Read the model definition and answer for the solid it produces. Units are mm, in the model's axes. Face numbers are marked on the shaded views. A direction names the side the tool comes from. Give positions to 0.01 mm unless a question says otherwise; leave off trailing zeros. Order: outer loops, then holes, each group sorted by start corner. A loop starts at its lowest first (then second) coordinate and runs counter-clockwise, first axis right, second up.
Item 1: A cutting plane is placed at B-B (y = 9.5). Write down the section's boundary in (x, z).
Item 2: A cutting plane is placed at A-A (x = 0). Write down the section's boundary in (y, z).
Item 3: The mould has two halves that part along X. Classify the marked faces 1 and 2: +X half, -X half, draft (parallel to the pull), parting line (faces both ways), or undercut.
Item 4: Find the intervals of material crossed by line 1 along Y through (x, z) = (0, 7.25); line 2 along X through (y, z) = (18.5, 7.75); line 3 along Y through (x, z) = (-77.5, 7.5), in increasing order.
Item 5: A cutting plane is placed at C-C (x = -61.5). Write down the section's boundary in (y, z).
Item 6: Given pin 1 Ø1 at (y, z) = (18.5, 1.5) entering from +X; pin 2 Ø1.5 at (x, z) = (-64.5, 6) entering from +Y; pin 3 Ø6 at (x, y) = (-5, 21.5) entering from -Z; pin 4 Ø6 at (x, y) = (-24.5, 15) entering from +Z, each flat-ended and moving along its own axis, determine where each tip first touches the part or whether it passes through.
Item 7: Which of the six approach directions +Z, -Z, +X, -X, +Y, -Y give full straight-line access (tool end or side, diameter ignored) to the marked faces 3 and 4?
Item 8: A cutting plane is placed at D-D (x = -104.5). Write down the section's boundary in (y, z), plus the area to 3 significant figures.
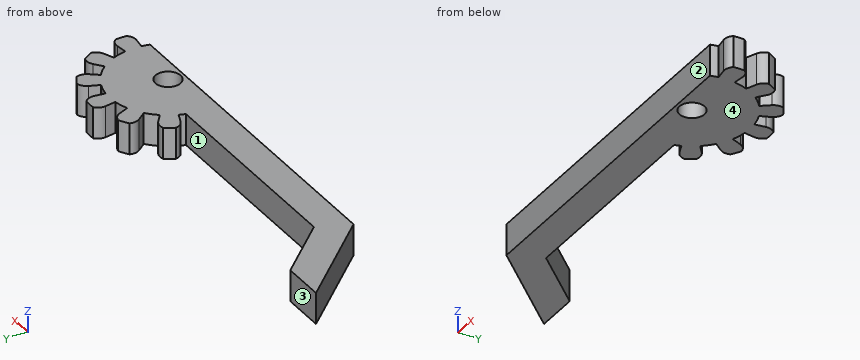
from build123d import *

# Parameters (mm, degrees)
SKETCH1_R           = 4
BOSS_EXTRUDE2_DEPTH = 10


with BuildPart() as part:
    # Sketch1 → Boss-Extrude2 (new body)
    with BuildSketch(Plane.XY):
        with BuildLine():
            Line((-101.371578153, 22), (-115, 22))
            Line((-115, 22), (-90, -5))
            Line((-90, -5), (17.811513131, -5))
            ThreePointArc((17.811513131, -5), (18.106389525, -3.79587386), (18.319959272, -2.574702368))
            Line((18.319959272, -2.574702368), (21.785897512, -3.061808221))
            ThreePointArc((21.785897512, -3.061808221), (23.533640729, -2.812333445), (24.939101256, -1.743911844))
            ThreePointArc((24.939101256, -1.743911844), (25, 0), (24.939101256, 1.743911844))
            ThreePointArc((24.939101256, 1.743911844), (23.533640729, 2.812333445), (21.785897512, 3.061808221))
            Line((21.785897512, 3.061808221), (18.319959272, 2.574702368))
            ThreePointArc((18.319959272, 2.574702368), (17.869627786, 4.788152334), (17.152901309, 6.930221978))
            Line((17.152901309, 6.930221978), (20.3980448, 8.241345055))
            ThreePointArc((20.3980448, 8.241345055), (21.786897437, 9.331268157), (22.469851157, 10.95927867))
            ThreePointArc((22.469851157, 10.95927867), (21.650635095, 12.5), (20.725939314, 13.979822587))
            ThreePointArc((20.725939314, 13.979822587), (18.974563992, 14.202372572), (17.336236579, 13.544552457))
            Line((17.336236579, 13.544552457), (14.578198942, 11.389737294))
            ThreePointArc((14.578198942, 11.389737294), (13.081475452, 13.081475452), (11.389737294, 14.578198942))
            Line((11.389737294, 14.578198942), (13.544552457, 17.336236579))
            ThreePointArc((13.544552457, 17.336236579), (14.202372572, 18.974563992), (13.979822587, 20.725939314))
            ThreePointArc((13.979822587, 20.725939314), (12.5, 21.650635095), (10.95927867, 22.469851157))
            ThreePointArc((10.95927867, 22.469851157), (9.331268157, 21.786897437), (8.241345055, 20.3980448))
            Line((8.241345055, 20.3980448), (6.930221978, 17.152901309))
            ThreePointArc((6.930221978, 17.152901309), (4.788152334, 17.869627786), (2.574702368, 18.319959272))
            Line((2.574702368, 18.319959272), (3.061808221, 21.785897512))
            ThreePointArc((3.061808221, 21.785897512), (2.812333445, 23.533640729), (1.743911844, 24.939101256))
            ThreePointArc((1.743911844, 24.939101256), (0, 25), (-1.743911844, 24.939101256))
            ThreePointArc((-1.743911844, 24.939101256), (-2.812333445, 23.533640729), (-3.061808221, 21.785897512))
            Line((-3.061808221, 21.785897512), (-2.574702368, 18.319959272))
            ThreePointArc((-2.574702368, 18.319959272), (-4.788152334, 17.869627786), (-6.930221978, 17.152901309))
            Line((-6.930221978, 17.152901309), (-8.241345055, 20.3980448))
            ThreePointArc((-8.241345055, 20.3980448), (-9.331268157, 21.786897437), (-10.95927867, 22.469851157))
            ThreePointArc((-10.95927867, 22.469851157), (-12.5, 21.650635095), (-13.979822587, 20.725939314))
            ThreePointArc((-13.979822587, 20.725939314), (-14.202372572, 18.974563992), (-13.544552457, 17.336236579))
            Line((-13.544552457, 17.336236579), (-11.389737294, 14.578198942))
            ThreePointArc((-11.389737294, 14.578198942), (-13.081475452, 13.081475452), (-14.578198942, 11.389737294))
            Line((-14.578198942, 11.389737294), (-17.336236579, 13.544552457))
            ThreePointArc((-17.336236579, 13.544552457), (-18.974563992, 14.202372572), (-20.725939314, 13.979822587))
            ThreePointArc((-20.725939314, 13.979822587), (-21.650635095, 12.5), (-22.469851157, 10.95927867))
            ThreePointArc((-22.469851157, 10.95927867), (-21.786897437, 9.331268157), (-20.3980448, 8.241345055))
            Line((-20.3980448, 8.241345055), (-17.152901309, 6.930221978))
            ThreePointArc((-17.152901309, 6.930221978), (-17.508826588, 5.974193795), (-17.811513131, 5))
            Line((-17.811513131, 5), (-85.630837413, 5))
            Line((-85.630837413, 5), (-101.371578153, 22))
        make_face()
        Circle(SKETCH1_R, mode=Mode.SUBTRACT)
    extrude(amount=BOSS_EXTRUDE2_DEPTH)


solid = part.part
Response values:
1. outline: (-103.43, 0) - (-89.8, 0) - (-89.8, 10) - (-103.43, 10) - close; (-21.91, 0) - (21.91, 0) - (21.91, 10) - (-21.91, 10) - close
2. outline: (-5, 0) - (-4, 0) - (-4, 10) - (-5, 10) - close; (4, 0) - (25, 0) - (25, 10) - (4, 10) - close
3. face 1: undercut
3. face 2: draft
4. line 1: y = -5 to -4, 4 to 25
4. line 2: x = -111.76 to -98.13, -14.11 to -7.47, -2.6 to 2.6, 7.47 to 14.11
4. line 3: y = -5 to 5
5. outline: (-5, 0) - (5, 0) - (5, 10) - (-5, 10) - close
6. pin 1: stops at x = 14.21
6. pin 2: stops at y = 5
6. pin 3: stops at z = 0
6. pin 4: passes through
7. face 3: +Z, -Z, -X, +Y
7. face 4: -Z, +X, -X, +Y, -Y
8. outline: (10.66, 0) - (22, 0) - (22, 10) - (10.66, 10) - close
8. area: 113 mm2
